Geometry check sheet. Reference: the model listing, model coordinates, mm. A direction names the side the tool comes from. Round coordinates to 2 decimals unless told otherwise and drop trailing zeros. Loops run counter-clockwise (first coordinate to the right, second up) from the corner with the lowest first, then second, coordinate; pieces in that order, holes last. Notation, with made-up numbers: (5.5, -12.75) -> (15.5, -12.75) arc R21 cw to (15.5, -4.75) -> close; hole circle Ø10 at (39.5, -28). An arc over 180 degrees is marked (long way). Use one line per item in the form item = value.
from build123d import *

# Parameters (mm, degrees)
SKETCH_1_R          = 2.25
EXTRUDE_1_DEPTH     = 2.5
CUT_EXTRUDE_1_DEPTH = 2
SKETCH_3_R          = 1.25
EXTRUDE_2_DEPTH     = 35
CHAMFER_1_SIZE      = 0.25


with BuildPart() as part:
    # 草图1 → 凸台-拉伸1 (new body)
    with BuildSketch(Plane(origin=(0, 0, 0), x_dir=(1, 0, 0), z_dir=(0, 1, 0))):
        with Locations(Location((0, 0, 0), (0, 0, 270))):
            Circle(SKETCH_1_R)
    extrude(amount=EXTRUDE_1_DEPTH)

    # 草图2 → 切除-拉伸1 (cut)
    with BuildSketch(Plane(origin=(0, 2.5, 0), x_dir=(1, 0, 0), z_dir=(0, 1, 0))):
        Polygon((0, 1.154700538), (-1, 0.577350269), (-1, -0.577350269), (0, -1.154700538), (1, -0.577350269), (1, 0.577350269), align=None)
    extrude(amount=-CUT_EXTRUDE_1_DEPTH, mode=Mode.SUBTRACT)

    # 草图3 → 凸台-拉伸2 (add)
    with BuildSketch(Plane.XZ):
        with Locations(Location((0, 0, 0), (0, 0, 270))):
            Circle(SKETCH_3_R)
    extrude(amount=EXTRUDE_2_DEPTH)

    # 倒角1
    chamfer_1_edges = [part.edges().sort_by_distance(p)[0] for p in [
        (0.5, 2.5, -0.866025404),
        (-0.5, 2.5, -0.866025404),
        (-1, 2.5, 0),
        (-0.5, 2.5, 0.866025404),
        (0.5, 2.5, 0.866025404),
        (1, 2.5, 0),
        (0, 0, -2.25),
        (0, -35, 1.25),
        (0, 2.5, -2.25),
    ]]
    chamfer(chamfer_1_edges, length=CHAMFER_1_SIZE)


solid = part.part
1. Section check A-A (z = 0). Record the boundary of the cut face in (x, y), then the cut area to 3 significant figures.
Return value:
outline = (-2.25, 0.25) -> (-2, 0) -> (-1.25, 0) -> (-1.25, -34.75) -> (-1, -35) -> (1, -35) -> (1.25, -34.75) -> (1.25, 0) -> (2, 0) -> (2.25, 0.25) -> (2.25, 2.25) -> (2, 2.5) -> (1.25, 2.5) -> (1, 2.25) -> (1, 0.5) -> (-1, 0.5) -> (-1, 2.25) -> (-1.25, 2.5) -> (-2, 2.5) -> (-2.25, 2.25) -> close
area = 94.5 mm2
2. Gauge pin test, flat ends, axial feed: pin 1 (1 mm diameter, centred on y = -25, z = -1.5, fed in from +X); pin 2 (2 mm diameter, centred on x = -0.5, z = -0.5, fed in from +Y); pin 3 (1.5 mm diameter, centred on y = -18, z = 0, fed in from +X). Record the tip position at first contact, or that the pin passes through.
Return value:
pin_1 = 0.75
pin_2 = 2.5
pin_3 = 1.25
3. Tool access check on faces 1 (the flat face through (0.57, 2.373, -0.968)), 2 (the flat face through (1, 0, 1)). Record the directions out of +Z, -Z, +X, -X, +Y, -Y that give a thin tool (end or side, any length) a straight path to the whole face; none if there is none.
Return value:
face_1 = +Y
face_2 = -Y
4. Section check B-B (y = -30). Record the boundary of the cut face in (x, z), then the cut area to 3 significant figures.
Return value:
outline = circle Ø2.5 at (0, 0)
area = 4.91 mm2
5. Material ranges on line 1 along X through (y, z) = (1, -0.1); line 2 along Y through (x, z) = (0.2, -1.55); line 3 along Y through (x, z) = (-0.45, -0.6), recorded low to high.
Return value:
line_1 = -2.25 to -1, 1 to 2.25
line_2 = 0 to 2.5
line_3 = -35 to 0.5
6. Mould release check, pull along Z, two halves, no side actions. Record for faces 3 (the flat face through (0, -35, 0)), 4 (the flat face through (0.553, 2.373, 0.978)), 5 (the cylindrical face through (0.676, 1.236, 2.146)): released by +Z, released by -Z, zero draft, split by the parting line, or undercut.
Return value:
face_3 = zero draft
face_4 = undercut
face_5 = split by the parting line
